The figure shows three views and two pictorial views of one solid part (mm, origin at its lowest corner). Answer the questions. A direction names the side the tool comes from. Coordinates: 2 decimals unless noted, no trailing zeros. Loops run counter-clockwise (first coordinate to the right, second up) from the corner with the lowest first, then second, coordinate; pieces in that order, holes last. Notation, with made-up numbers: (-10.5, 13.5) -> (19.5, 13.5) arc R16 cw to (19.5, 26.5) -> close; hole circle Ø2 at (62.5, 70). An arc over 180 degrees is marked (long way). Answer as a JSON object with one key per item and string values. Group by question number.
1) Section B-B, the plane y = 7.5 is taken. Give the vertices of the cut face in (x, z) (3 decimals).
2) Consider probe 1 along Y at (x, z) = (7.5, 22.8); probe 2 along Z at (x, y) = (7.5, 2.5) (3 decimals); probe 3 along Y at (x, z) = (11, 9) (3 decimals). Determine where each line is inside the solid, lowest interval first. Write a range as [from, to].
3) Section C-C, the plane z = 5 is taken. Give the vertices of the cut face in (x, y) (3 decimals), plus the area to 3 significant figures.
4) Section D-D, the plane y = 12.25 is taken. Give the vertices of the cut face in (x, z) (3 decimals).
5) Determine the mould class of the marked faces 3, 4 and 5 for opening direction Z: released by +Z, released by -Z, zero draft, split by the parting line, or undercut.
6) Flat-ended cylindrical pins translate along their axes: P1, Ø6, axis at x = 8.5, y = 7.5, coming from the -Z side; P2, Ø5, axis at x = 8.5, z = 15.5, coming from the -Y side (3 decimals); P3, Ø3.5, axis at x = 7.5, z = 7.5, coming from the +Y side. Find the tip coordinate at first contact, or state that the pin passes through.
7) Section A-A, the plane x = 7.5 is taken. Give the vertices of the cut face in (y, z) (3 decimals), plus the area to 3 significant figures.
8) Which of the six approach directions +Z, -Z, +X, -X, +Y, -Y give full straight-line access (tool end or side, diameter ignored) to the marked faces 1 and 2?
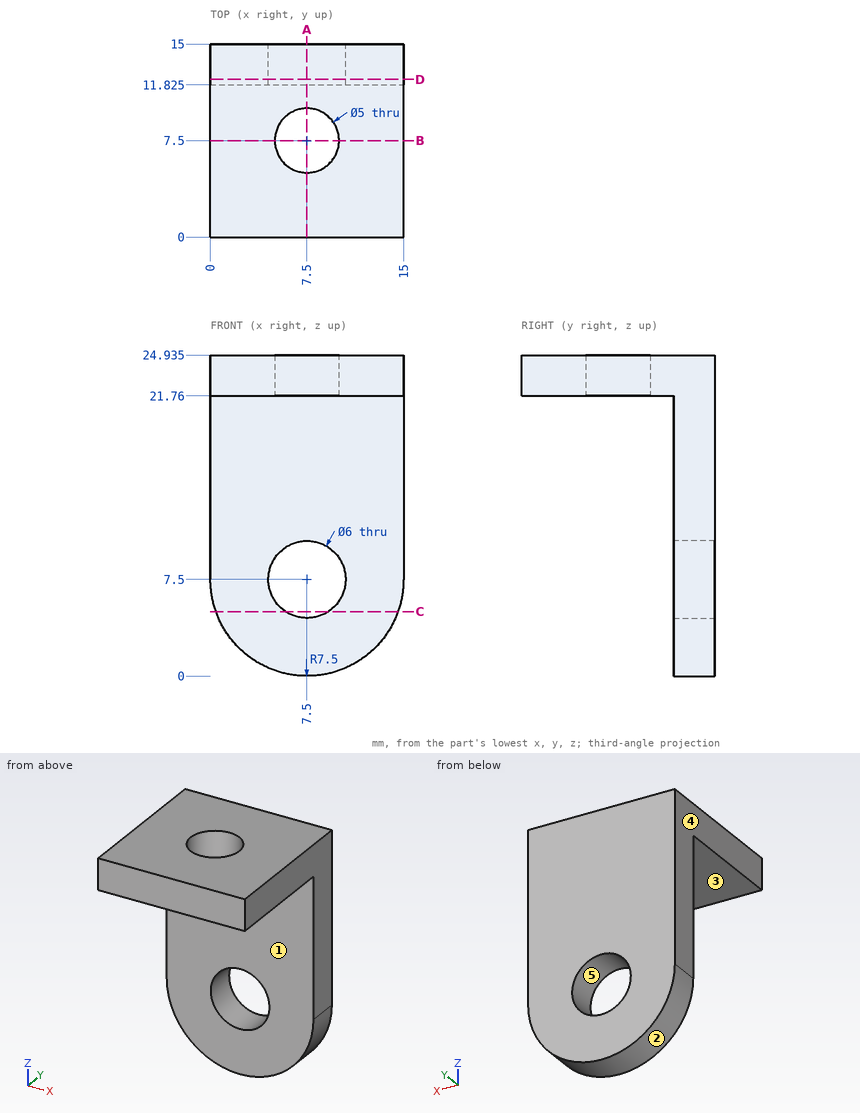
Determined:
{
 "1": {"outline": "(0, 21.76) -> (5, 21.76) -> (5, 24.935) -> (0, 24.935) -> close; (10, 21.76) -> (15, 21.76) -> (15, 24.935) -> (10, 24.935) -> close"},
 "2": {"probe 1": "[0, 5], [10, 15]", "probe 2": "[21.76, 24.935]", "probe 3": "[11.825, 15]"},
 "3": {"outline": "(0.429, 11.825) -> (5.842, 11.825) -> (5.842, 15) -> (0.429, 15) -> close; (9.158, 11.825) -> (14.571, 11.825) -> (14.571, 15) -> (9.158, 15) -> close", "area": "34.4 mm²"},
 "4": {"outline": "(0, 7.5) arc R7.5 ccw to (15, 7.5) -> (15, 24.935) -> (0, 24.935) -> close; hole circle Ø6 at (7.5, 7.5)"},
 "5": {"face 3": "released by -Z", "face 4": "zero draft", "face 5": "undercut"},
 "6": {"P1": "z = 21.76", "P2": "y = 11.825", "P3": "through"},
 "7": {"outline": "(0, 21.76) -> (5, 21.76) -> (5, 24.935) -> (0, 24.935) -> close; (10, 21.76) -> (11.825, 21.76) -> (11.825, 10.5) -> (15, 10.5) -> (15, 24.935) -> (10, 24.935) -> close; (11.825, 0) -> (15, 0) -> (15, 4.5) -> (11.825, 4.5) -> close", "area": "81.8 mm²"},
 "8": {"face 1": "-Z, +X, -X, -Y", "face 2": "-Z, +Y, -Y"}
}
